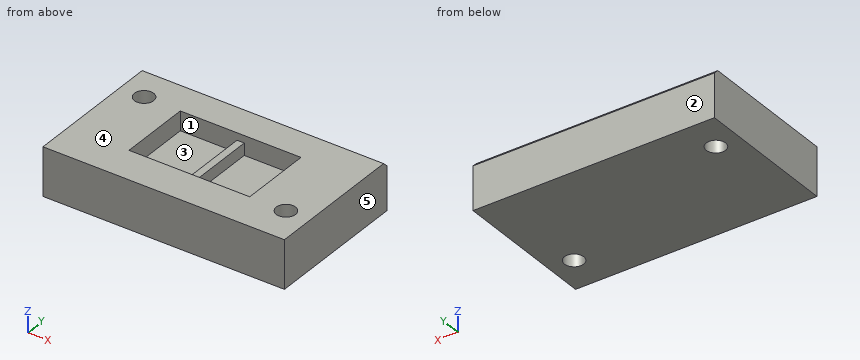
```python
from build123d import *

# Parameters (mm, degrees)
SKIZZE1_W                       = 100
SKIZZE1_H                       = 60
AUFSATZ_LINEAR_AUSTRAGEN1_DEPTH = 20
SKIZZE2_W                       = 50
SKIZZE2_H                       = 30
SCHNITT_LINEAR_AUSTRAGEN1_DEPTH = 8
SKIZZE3_R                       = 4
SCHNITT_LINEAR_AUSTRAGEN2_DEPTH = 62.64414003
SKIZZE4_R                       = 4
SCHNITT_LINEAR_AUSTRAGEN3_DEPTH = 62.64414003
VERST_RKUNGSRIPPE1_START        = -1.5
VERST_RKUNGSRIPPE1_OUTLINE_W    = 5
VERST_RKUNGSRIPPE1_OUTLINE_H    = 30
VERST_RKUNGSRIPPE1_DEPTH        = 3
FASE1_SIZE                      = 2


# Read off the part's stored shape, not the designer's step: Verst_rkungsrippe1
with BuildPart() as part:
    # Skizze1 → Aufsatz-Linear austragen1 (new body)
    with BuildSketch(Plane.XY):
        Rectangle(SKIZZE1_W, SKIZZE1_H)
    extrude(amount=AUFSATZ_LINEAR_AUSTRAGEN1_DEPTH)

    # Skizze2 → Schnitt-Linear austragen1 (cut)
    with BuildSketch(Plane.XY.offset(20)):
        Rectangle(SKIZZE2_W, SKIZZE2_H)
    extrude(amount=-SCHNITT_LINEAR_AUSTRAGEN1_DEPTH, mode=Mode.SUBTRACT)

    # Skizze3 → Schnitt-Linear austragen2 (cut, through all)
    with BuildSketch(Plane.XY.offset(20)):
        with Locations((-40, 15)):
            Circle(SKIZZE3_R)
    extrude(amount=-SCHNITT_LINEAR_AUSTRAGEN2_DEPTH, mode=Mode.SUBTRACT)

    # Skizze4 → Schnitt-Linear austragen3 (cut, through all)
    with BuildSketch(Plane.XY.offset(20)):
        with Locations((40, -15)):
            Circle(SKIZZE4_R)
    extrude(amount=-SCHNITT_LINEAR_AUSTRAGEN3_DEPTH, mode=Mode.SUBTRACT)

    # Verst_rkungsrippe1 outline → Verst_rkungsrippe1 (add)
    with BuildSketch(Plane(origin=(0, 0, 0), x_dir=(0, 0, -1), z_dir=(1, 0, 0)).offset(VERST_RKUNGSRIPPE1_START)):
        with Locations((-14.5, 0)):
            Rectangle(VERST_RKUNGSRIPPE1_OUTLINE_W, VERST_RKUNGSRIPPE1_OUTLINE_H)
    extrude(amount=VERST_RKUNGSRIPPE1_DEPTH)

    # Fase1
    fase1_edges = [part.edges().sort_by_distance(p)[0] for p in [
        (0, 30, 20),
    ]]
    chamfer(fase1_edges, length=FASE1_SIZE)


solid = part.part
```
Can you work these out from the model? Positions are in its coordinate system, mm. Face numbers are marked on the shaded views. A direction names the side the tool comes from. Give positions to 0.01 mm unless a question says otherwise; leave off trailing zeros. Order: outer loops, then holes, each group sorted by start corner. A loop starts at its lowest first (then second) coordinate and runs counter-clockwise, first axis right, second up. Notation, with made-up numbers: M 79.25,27 L 124.25,27 A36 ccw 124.25,66 Z; hole C 28.25,-37.75 d6. An arc over 180 degrees is marked long. Write item = value, one per line. Start each with the question number.
Q1. For the marked faces 1 and 2, which set-ups out of +Z, -Z, +X, -X, +Y, -Y let a thin tool reach every point of the face, with its end or its side?
Q2. We'd pull the mould along X, two halves only. Please class the marked faces 3, 4 and 5: pulls with the +X half, pulls with the -X half, needs draft (parallel to the pull), parting line crosses it, or undercut.
Q3. Suppose I cut it at C-C (x = 8.5). Write out the boundary of the cut face in (y, z).
Q4. Suppose I cut it at A-A (z = 13.5). Write out the boundary of the cut face in (x, y), plus the area to 3 significant figures.
Q5. Suppose I cut it at D-D (y = 3). Write out the boundary of the cut face in (x, z), plus the area to 4 significant figures.
Q6. I need wall thicknesses on probe 1 along X at (y, z) = (-2, 12.75); probe 2 along Y at (x, z) = (40, 5.75); probe 3 along Y at (x, z) = (18, 16.25). Which ranges of each line are inside material? Lowest first, please. Write a range as [from, to].
Q7. Will these pins go through, and if not, where does the flat tip stop? pin 1 Ø3.5 at (x, y) = (-0.5, 6.5) entering from +Z; pin 2 Ø7 at (x, y) = (14, 0.5) entering from +Z.
Q8. Suppose I cut it at B-B (x = -40). Write out the boundary of the cut face in (y, z).
Check result:
q1.face_1 = +Z
q1.face_2 = +Z, -Z, +X, -X, +Y
q2.face_3 = undercut
q2.face_4 = needs draft
q2.face_5 = pulls with the +X half
q3.outline = M -30,0 L 30,0 L 30,18 L 28,20 L 15,20 L 15,12 L -15,12 L -15,20 L -30,20 Z
q4.outline = M -50,-30 L 50,-30 L 50,30 L -50,30 Z; hole C -40,15 d8; hole M -25,-15 L -1.5,-15 L -1.5,15 L -25,15 Z; hole M 1.5,-15 L 25,-15 L 25,15 L 1.5,15 Z; hole C 40,-15 d8
q4.area = 4,490 mm2
q5.outline = M -50,0 L 50,0 L 50,20 L 25,20 L 25,12 L 1.5,12 L 1.5,17 L -1.5,17 L -1.5,12 L -25,12 L -25,20 L -50,20 Z
q5.area = 1,615 mm2
q6.probe_1 = [-50, -25], [-1.5, 1.5], [25, 50]
q6.probe_2 = [-30, -19], [-11, 30]
q6.probe_3 = [-30, -15], [15, 30]
q7.pin_1 = 17
q7.pin_2 = 12
q8.outline = M -30,0 L 11,0 L 11,20 L -30,20 Z; M 19,0 L 30,0 L 30,18 L 28,20 L 19,20 Z
